Verification items for the finished model (mm, model axes). Face numbers are marked on the shaded views. Round coordinates to 2 decimals unless told otherwise and drop trailing zeros. Order: outer loops, then holes, each group sorted by start corner. A loop starts at its lowest first (then second) coordinate and runs counter-clockwise, first axis right, second up. Notation, with made-up numbers: (13, 40) -> (18, 40) arc R25 cw to (18, 77) -> close; hole circle Ø5 at (-25.75, 59.5). An arc over 180 degrees is marked (long way). Return JSON: item names as keys, results as strings. Group by question number.
1) Section check D-D on y = 9.75. Enter the section's corners in (x, z).
2) Section check B-B on y = 5. Enter the section's corners in (x, z), plus the area to 3 significant figures.
3) Section check A-A on x = 6.5. Enter the section's corners in (y, z).
4) Draft check along Z on the marked faces 1, 2, 3 and 4. Enter one of: pulls with the +Z half, pulls with the -Z half, needs draft (parallel to the pull), parting line crosses it, or undercut.
5) Section check C-C on z = -10. Enter the section's corners in (x, y).
6) Scan lines: L1, parallel to Y at x = 9, z = 10; L2, parallel to Z at x = 8.75, y = 6; L3, parallel to X at y = 8.75, z = 1. Record each from-to range of solid material in increasing order.
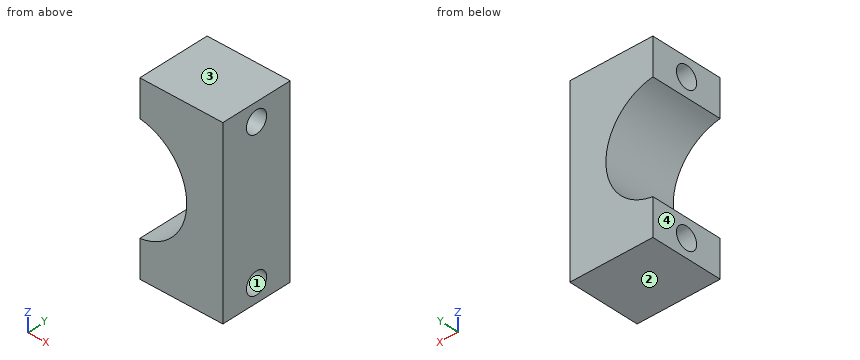
```python
from build123d import *

# Parameters (mm, degrees)
SKETCH1_W           = 25
SKETCH1_H           = 25
BOSS_EXTRUDE1_DEPTH = 10
SKETCH2_R           = 7.5
CUT_EXTRUDE1_DEPTH  = 21.310096012
SKETCH3_W           = 12.5
SKETCH3_H           = 25
CUT_EXTRUDE2_DEPTH  = 10
SKETCH4_R           = 1.5
CUT_EXTRUDE3_DEPTH  = 21.310096012
CUT_EXTRUDE4_DEPTH  = 21.310096012


with BuildPart() as part:
    # Sketch1 → Boss-Extrude1 (new body)
    with BuildSketch(Plane(origin=(0, 0, 0), x_dir=(1, 0, 0), z_dir=(0, 1, 0))):
        Rectangle(SKETCH1_W, SKETCH1_H)
    extrude(amount=BOSS_EXTRUDE1_DEPTH)

    # Sketch2 → Cut-Extrude1 (cut, through all)
    with BuildSketch(Plane(origin=(0, 10, 0), x_dir=(1, 0, 0), z_dir=(0, 1, 0))):
        with Locations(Location((0, 0, 0), (0, 0, 270))):
            Circle(SKETCH2_R)
    extrude(amount=-CUT_EXTRUDE1_DEPTH, mode=Mode.SUBTRACT)

    # Sketch3 → Cut-Extrude2 (cut)
    with BuildSketch(Plane(origin=(0, 10, 0), x_dir=(1, 0, 0), z_dir=(0, 1, 0))):
        with Locations((-6.25, 0)):
            Rectangle(SKETCH3_W, SKETCH3_H)
    extrude(amount=-CUT_EXTRUDE2_DEPTH, mode=Mode.SUBTRACT)

    # Sketch4 → Cut-Extrude3 (cut, through all)
    with BuildSketch(Plane.ZY):
        with Locations((-10, 5)):
            Circle(SKETCH4_R)
        with Locations((10, 5)):
            Circle(SKETCH4_R)
    extrude(amount=-CUT_EXTRUDE3_DEPTH, mode=Mode.SUBTRACT)

    # Sketch5 → Cut-Extrude4 (cut, through all)
    with BuildSketch(Plane(origin=(0, 10, 0), x_dir=(1, 0, 0), z_dir=(0, 1, 0))):
        with BuildLine():
            Line((1, 12.5), (0, 12.5))
            Line((0, 12.5), (0, 7.5))
            ThreePointArc((0, 7.5), (0.501119845, 7.483239867), (1, 7.433034374))
            Line((1, 7.433034374), (1, 12.5))
        make_face()
        with BuildLine():
            ThreePointArc((1, -7.433034374), (0.501119845, -7.483239867), (0, -7.5))
            Line((0, -7.5), (0, -12.5))
            Line((0, -12.5), (1, -12.5))
            Line((1, -12.5), (1, -7.433034374))
        make_face()
        with BuildLine():
            ThreePointArc((1, 7.433034374), (0.501119845, 7.483239867), (0, 7.5))
            Line((0, 7.5), (0, -7.5))
            ThreePointArc((0, -7.5), (0.501119845, -7.483239867), (1, -7.433034374))
            Line((1, -7.433034374), (1, 7.433034374))
        make_face()
    extrude(amount=-CUT_EXTRUDE4_DEPTH, mode=Mode.SUBTRACT)


solid = part.part
```
Check result:
{
 "1": {"outline": "(1, -12.5) -> (12.5, -12.5) -> (12.5, 12.5) -> (1, 12.5) -> (1, 7.43) arc R7.5 cw to (1, -7.43) -> close"},
 "2": {"outline": "(1, -12.5) -> (12.5, -12.5) -> (12.5, -11.5) -> (1, -11.5) -> close; (1, -8.5) -> (12.5, -8.5) -> (12.5, 8.5) -> (1, 8.5) -> (1, 7.43) arc R7.5 cw to (1, -7.43) -> close; (1, 11.5) -> (12.5, 11.5) -> (12.5, 12.5) -> (1, 12.5) -> close", "area": "145 mm^2"},
 "3": {"outline": "(0, -12.5) -> (10, -12.5) -> (10, -3.74) -> (0, -3.74) -> close; (0, 3.74) -> (10, 3.74) -> (10, 12.5) -> (0, 12.5) -> close; hole circle Ø3 at (5, -10); hole circle Ø3 at (5, 10)"},
 "4": {"face 1": "undercut", "face 2": "pulls with the -Z half", "face 3": "pulls with the +Z half", "face 4": "needs draft"},
 "5": {"outline": "(1, 0) -> (12.5, 0) -> (12.5, 3.5) -> (1, 3.5) -> close; (1, 6.5) -> (12.5, 6.5) -> (12.5, 10) -> (1, 10) -> close"},
 "6": {"L1": "0 to 3.5, 6.5 to 10", "L2": "-12.5 to -11.12, -8.88 to 8.88, 11.12 to 12.5", "L3": "7.43 to 12.5"}
}
